Geometry: final body of the model. Coordinates: model frame, mm. A direction names the side the tool comes from. Coordinates: 2 decimals unless noted, no trailing zeros. Loops run counter-clockwise (first coordinate to the right, second up) from the corner with the lowest first, then second, coordinate; pieces in that order, holes last. Notation, with made-up numbers: (22.25, 44.5) - (34.25, 44.5) arc R23 cw to (34.25, 65.5) - close; hole circle Ø7 at (-22.5, -7.75). An arc over 180 degrees is marked (long way). Put each result on its own line as item: value. Start each with the question number.
1) Reachability of faces 1 (the flat face through (4.35, 26.451, -2.465)), 2 (the flat face through (5, 30, -2)), 3 (the cylindrical face through (-0.867, 9.86, 3.905)) from +Z, -Z, +X, -X, +Y, -Y: full face, straight path, thin tool, end or side. Return the list, or none.
2) Section C-C on z = -2.25. Output: boundary loops of the cut face in (x, y), and give its area (3 significant figures).
3) Material intervals for line 1 along Z through (x, y) = (0, 27); line 2 along Y through (x, z) = (3, 4.25); line 3 along Y through (x, z) = (-3.25, -5.25), sorted ascending. Write a range as from..to.
4) Section D-D on x = -5. Output: boundary loops of the cut face in (y, z).
5) Section B-B on x = 0. Output: boundary loops of the cut face in (y, z), and give its area (3 significant figures).
6) Section A-A on y = 27.25. Output: boundary loops of the cut face in (x, z).
7) Draft query along X for faces 4 (the cylindrical face through (-7.493, 24.93, -0.33)), 5 (the flat face through (-4.31, 26.451, -2.535)), 6 (the flat face through (0, 0, 0)). Return one class per face: +X half, -X half, draft (parallel to the pull), parting line (faces both ways), or undercut.
8) Contact query for flat-ended pins moving along their axis: pin 1 Ø4 at (y, z) = (12.5, -3.5) entering from -X; pin 2 Ø2 at (x, y) = (-4.5, 8) entering from +Z; pin 3 Ø1 at (x, z) = (3, 1.5) entering from +Y. Output: stop coordinate, or through.
```python
from build123d import *

# Parameters (mm, degrees)
SKETCH1_R           = 4
BOSS_EXTRUDE1_DEPTH = 20
SKETCH2_R           = 7.5
BOSS_EXTRUDE2_DEPTH = 3
SKETCH3_R           = 7.5
BOSS_EXTRUDE3_DEPTH = 7


with BuildPart() as part:
    # Sketch1 → Boss-Extrude1 (new body)
    with BuildSketch(Plane(origin=(0, 0, 0), x_dir=(1, 0, 0), z_dir=(0, 1, 0))):
        Circle(SKETCH1_R)
    extrude(amount=BOSS_EXTRUDE1_DEPTH)

    # Sketch2 → Boss-Extrude2 (add)
    with BuildSketch(Plane(origin=(0, 20, 0), x_dir=(1, 0, 0), z_dir=(0, 1, 0))):
        Circle(SKETCH2_R)
    extrude(amount=BOSS_EXTRUDE2_DEPTH)

    # Sketch3 → Boss-Extrude3 (add)
    with BuildSketch(Plane(origin=(0, 23, 0), x_dir=(1, 0, 0), z_dir=(0, 1, 0))):
        Circle(SKETCH3_R)
        Polygon((5.773502692, 0), (2.886751346, 5), (-2.886751346, 5), (-5.773502692, 0), (-2.886751346, -5), (2.886751346, -5), align=None, mode=Mode.SUBTRACT)
    extrude(amount=BOSS_EXTRUDE3_DEPTH)


solid = part.part
```
Answer block:
1. face 1: +Y
1. face 2: +Z, -Z, +X, -X, +Y
1. face 3: -Y
2. outline: (-7.15, 20) - (-3.31, 20) - (-3.31, 0) - (3.31, 0) - (3.31, 20) - (7.15, 20) - (7.15, 30) - (4.47, 30) - (4.47, 23) - (-4.47, 23) - (-4.47, 30) - (-7.15, 30) - close
2. area: 213 mm²
3. line 1: z = -7.5..-5, 5..7.5
3. line 2: y = 20..23
3. line 3: y = 20..30
4. outline: (20, -5.59) - (30, -5.59) - (30, -1.34) - (23, -1.34) - (23, 1.34) - (30, 1.34) - (30, 5.59) - (20, 5.59) - close
5. outline: (0, -4) - (20, -4) - (20, -7.5) - (30, -7.5) - (30, -5) - (23, -5) - (23, 5) - (30, 5) - (30, 7.5) - (20, 7.5) - (20, 4) - (0, 4) - close
5. area: 240 mm²
6. outline: circle Ø15 at (0, 0); hole (-5.77, 0) - (-2.89, -5) - (2.89, -5) - (5.77, 0) - (2.89, 5) - (-2.89, 5) - close
7. face 4: parting line
7. face 5: undercut
7. face 6: draft
8. pin 1: stops at x = -3.71
8. pin 2: stops at z = 1.94
8. pin 3: stops at y = 23
